Source: CAD feature listing. Evaluate the final solid. Frame: model axes, mm. A direction names the side the tool comes from. Give positions to 0.01 mm unless a question says otherwise; leave off trailing zeros. Answer in a Markdown table with one row per item. Add a question column.
(1) Pin query (flat end, axial travel): P1, Ø5, axis at y = 8.5, z = -9, coming from the +X side; P2, Ø4, axis at y = 19, z = 8.5, coming from the +X side; P3, Ø8, axis at y = 10, z = 3, coming from the -X side; P4, Ø1, axis at x = -1, z = -18.5, coming from the +Y side. Return the tip coordinate at first contact, or that it passes through.
(2) Mould query, pull axis Y, two halves, no side actions, for faces 1 (the face through (0.01, -6.8, -11.78)), 2 (the face through (0.004, -5.961, -26.846)). Classes: pulls with the +Y half, pulls with the -Y half, needs draft (parallel to the pull), parting line crosses it, or undercut.
(3) Set-up query: faces 3 (the face through (-1, 5, 0)), 4 (the face through (0.01, 6.3, 6.21)). Return all of +Z, -Z, +X, -X, +Y, -Y with unobstructed straight access to the full face (end or side cutting, diameter ignored); none if empty.
(4) Material intervals for line 1 along Y through (x, z) = (0.7, 2); line 2 along Z through (x, y) = (-0.45, 7); line 3 along Z through (x, y) = (-0.4, 10), sorted ascending.
from build123d import *

# Parameters (mm, degrees)
F0_R     = 24.5
F0_R_2   = 3
F1_DEPTH = 1
F0_R_3   = 27.5
F2_DEPTH = 1.75
F3_R     = 1.5
F5_R     = 3


# Not quite as in the source:
# - a fillet or chamfer that OpenCascade refuses, or shapes differently, is made with other operations: its cross-section is extruded or revolved along the edge and cut away or added


with BuildPart() as f1:
    # F0 (on Right) → F1 (new body, symmetric)
    with BuildSketch(Plane.YZ):
        Circle(F0_R)
        with BuildLine():
            ThreePointArc((0, 18.9637232794), (13.4093773274, 13.4093773274), (18.9637232794, 0))
            ThreePointArc((18.9637232794, 0), (18.3175500781, -4.9081727508), (16.4230661103, -9.4818616397))
            ThreePointArc((16.4230661103, -9.4818616397), (4.9081727508, -18.3175500781), (-9.4818616397, -16.4230661103))
            ThreePointArc((-9.4818616397, -16.4230661103), (-13.4093773274, -13.4093773274), (-16.4230661103, -9.4818616397))
            ThreePointArc((-16.4230661103, -9.4818616397), (-18.3175500781, 4.9081727508), (-9.4818616397, 16.4230661103))
            ThreePointArc((-9.4818616397, 16.4230661103), (-4.9081727508, 18.3175500781), (0, 18.9637232794))
        make_face(mode=Mode.SUBTRACT)
        with BuildLine():
            ThreePointArc((7.6604867484, -4.4227840863), (8.5441627462, -2.2894015078), (8.8455681727, 0))
            ThreePointArc((8.8455681727, 0), (6.2547612383, 6.2547612383), (0, 8.8455681727))
            ThreePointArc((0, 8.8455681727), (-2.2894015078, 8.5441627462), (-4.4227840863, 7.6604867484))
            ThreePointArc((-4.4227840863, 7.6604867484), (-8.5441627462, 2.2894015078), (-7.6604867484, -4.4227840863))
            ThreePointArc((-7.6604867484, -4.4227840863), (-6.2547612383, -6.2547612383), (-4.4227840863, -7.6604867484))
            ThreePointArc((-4.4227840863, -7.6604867484), (2.2894015078, -8.5441627462), (7.6604867484, -4.4227840863))
        make_face()
        Circle(F0_R_2, mode=Mode.SUBTRACT)
        with BuildLine():
            Line((0, 8.8455681727), (0, 18.9637232794))
            ThreePointArc((0, 18.9637232794), (-4.9081727508, 18.3175500781), (-9.4818616397, 16.4230661103))
            Line((-9.4818616397, 16.4230661103), (-4.4227840863, 7.6604867484))
            ThreePointArc((-4.4227840863, 7.6604867484), (-2.2894015078, 8.5441627462), (0, 8.8455681727))
        make_face()
        with BuildLine():
            ThreePointArc((-16.4230661103, -9.4818616397), (-13.4093773274, -13.4093773274), (-9.4818616397, -16.4230661103))
            Line((-9.4818616397, -16.4230661103), (-4.4227840863, -7.6604867484))
            ThreePointArc((-4.4227840863, -7.6604867484), (-6.2547612383, -6.2547612383), (-7.6604867484, -4.4227840863))
            Line((-7.6604867484, -4.4227840863), (-16.4230661103, -9.4818616397))
        make_face()
        with BuildLine():
            ThreePointArc((16.4230661103, -9.4818616397), (18.3175500781, -4.9081727508), (18.9637232794, 0))
            Line((18.9637232794, 0), (8.8455681727, 0))
            ThreePointArc((8.8455681727, 0), (8.5441627462, -2.2894015078), (7.6604867484, -4.4227840863))
            Line((7.6604867484, -4.4227840863), (16.4230661103, -9.4818616397))
        make_face()
    extrude(amount=F1_DEPTH, both=True)

    # F0 (on Right) → F2 (join, symmetric)
    with BuildSketch(Plane.YZ):
        Circle(F0_R_3)
        Circle(F0_R, mode=Mode.SUBTRACT)
    extrude(amount=F2_DEPTH, both=True)

    # F3
    f3_edges = [f1.edges().sort_by_distance(p)[0] for p in [
        (-1.75, -27.5, 0),
        (1.75, -27.5, 0),
    ]]
    fillet(f3_edges, radius=F3_R)

    # F4: fillet of radius 1 on 2 edges, made by hand

    # F4_s1 → F4_t2 (revolve, cut)
    with BuildSketch(Plane.XY):
        with BuildLine():
            ThreePointArc((1.75, 25.4682458366), (1.540569415, 24.8558734009), (1, 24.5))
            Line((1, 24.5), (1.75, 24.5))
            Line((1.75, 24.5), (1.75, 25.4682458366))
        make_face()
    revolve(axis=Axis((1.75, 0, 0), (1, 0, 0)), mode=Mode.SUBTRACT)

    # F4_s3 → F4_t4 (revolve, cut)
    with BuildSketch(Plane.XY):
        with BuildLine():
            ThreePointArc((-1.75, 25.4682458366), (-1.540569415, 24.8558734009), (-1, 24.5))
            Line((-1, 24.5), (-1.75, 24.5))
            Line((-1.75, 24.5), (-1.75, 25.4682458366))
        make_face()
    revolve(axis=Axis((-1.75, 0, 0), (1, 0, 0)), mode=Mode.SUBTRACT)

    # F5
    f5_edges = [f1.edges().sort_by_distance(p)[0] for p in [
        (0, -16.423066, -9.481862),
        (0, -7.660487, -4.422784),
        (0, -4.422784, 7.660487),
        (0, 0, 18.963723),
        (0, -9.481862, 16.423066),
        (0, -4.422784, -7.660487),
        (0, 7.660487, -4.422784),
        (0, 0, 8.845568),
        (0, 8.845568, 0),
        (0, -9.481862, -16.423066),
        (0, 16.423066, -9.481862),
        (0, 18.963723, 0),
    ]]
    fillet(f5_edges, radius=F5_R)


solid = f1.part
Values follow:
| question | item | result |
|---|---|---|
| 1 | P1 | passes through |
| 1 | P2 | stops at x = 1 |
| 1 | P3 | stops at x = -1 |
| 1 | P4 | stops at y = 20.62 |
| 2 | face 1 | undercut |
| 2 | face 2 | parting line crosses it |
| 3 | face 3 | -X |
| 3 | face 4 | +X, -X |
| 4 | line 1 | y = -27.36 to -18.86, -8.62 to -2.24, 2.24 to 8.63, 18.51 to 27.36 |
| 4 | line 2 | z = -26.58 to -17.62, -5.69 to 5.41, 17.62 to 26.58 |
| 4 | line 3 | z = -25.61 to -16.11, -5.77 to 0.38, 16.11 to 25.61 |
